The figure shows three views and two pictorial views of one solid part (mm, origin at its lowest corner). Answer the questions. A direction names the side the tool comes from. Round coordinates to 2 decimals unless told otherwise and drop trailing zeros. Loops run counter-clockwise (first coordinate to the right, second up) from the corner with the lowest first, then second, coordinate; pieces in that order, holes last. Notation, with made-up numbers: (40.5, -31.75) - (89.5, -31.75) arc R29 cw to (89.5, 0.25) - close; hole circle Ø2 at (-1.75, 7.5). An arc over 180 degrees is marked (long way). Use one line per item in the form item = value. Start each with the question number.
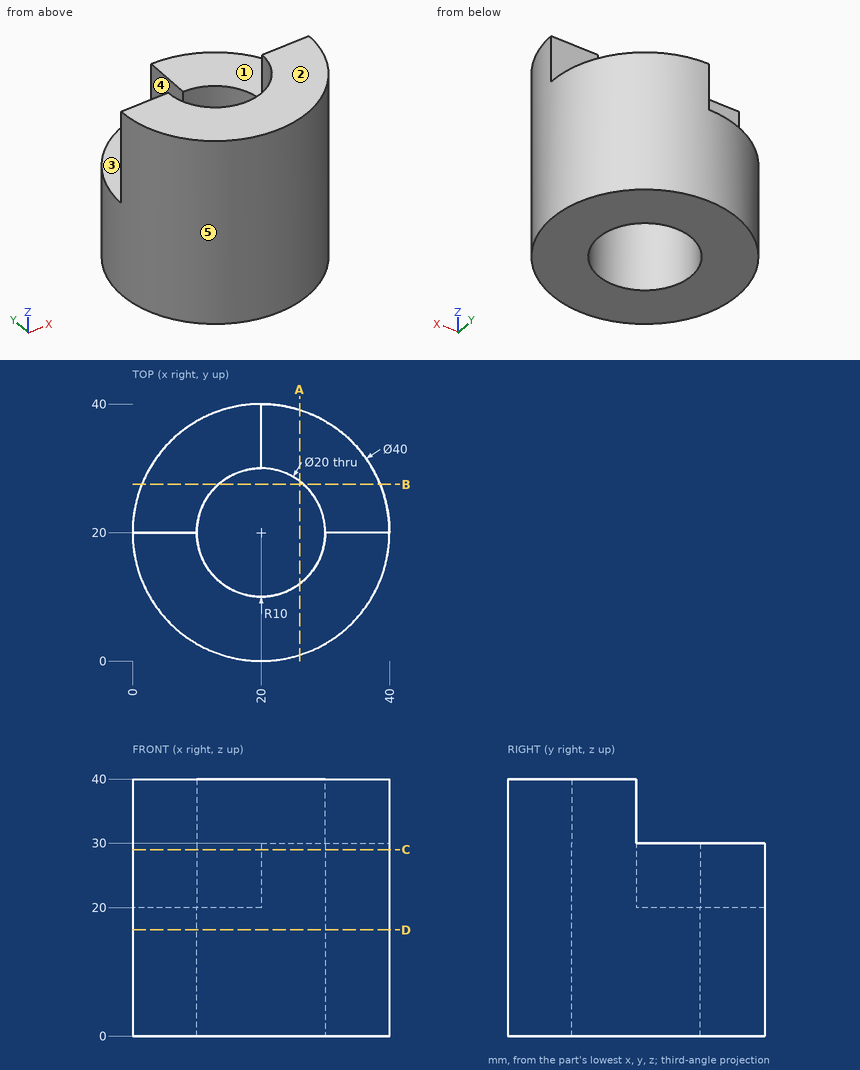
1) Straight lines are drawn through the part: line 1 (X direction, y = 20, z = 12.25); line 2 (Y direction, x = 13.5, z = 9.5). For each, find the intervals that lie inside material, in ascending order. Write a range as from..to.
2) A cutting plane is placed at B-B on y = 27.5. Write down the section's boundary in (x, z).
3) A cutting plane is placed at A-A on x = 26. Write down the section's boundary in (y, z), plus the area to 3 significant figures.
4) For the marked faces 1 and 2, determine the directions among +Z, -Z, +X, -X, +Y, -Y from which every point of the face is accessible in a straight line to the end or side of a thin tool.
5) Flat-ended cylindrical pins translate along their axes: pin 1 (5 mm diameter, centred on x = 4.5, z = 33.5, fed in from +Y); pin 2 (1 mm diameter, centred on x = 32, z = 13.5, fed in from -Y); pin 3 (5 mm diameter, centred on y = 33, z = 25.5, fed in from -X); pin 4 (1.5 mm diameter, centred on x = 26.5, y = 25.5, fed in from +Z). Find the tip coordinate at first contact, or state that the pin passes through.
6) A cutting plane is placed at D-D on z = 16.5. Write down the section's boundary in (x, y).
7) Determine the mould class of the marked faces 3, 4 and 5 for opening direction X: +X half, -X half, draft (parallel to the pull), parting line (faces both ways), or undercut.
8) A cutting plane is placed at C-C on z = 29. Write down the section's boundary in (x, y), plus the area to 3 significant figures.
Checks:
q1.line_1 = 0..10, 30..40
q1.line_2 = 1.09..12.4, 27.6..38.91
q2.outline = (1.46, 0) - (13.39, 0) - (13.39, 20) - (1.46, 20) - close; (26.61, 0) - (38.54, 0) - (38.54, 30) - (26.61, 30) - close
q3.outline = (0.92, 0) - (12, 0) - (12, 40) - (0.92, 40) - close; (28, 0) - (39.08, 0) - (39.08, 30) - (28, 30) - close
q3.area = 776 mm²
q4.face_1 = +Z, +X, -X, +Y
q4.face_2 = +Z, +X, -X, +Y, -Y
q5.pin_1 = 20
q5.pin_2 = 3.64
q5.pin_3 = 20
q5.pin_4 = through
q6.outline = circle Ø40 at (20, 20); hole circle Ø20 at (20, 20)
q7.face_3 = draft
q7.face_4 = -X half
q7.face_5 = parting line
q8.outline = (0, 20) arc R20 ccw (long way) to (20, 40) - (20, 30) arc R10 cw (long way) to (10, 20) - close
q8.area = 707 mm²
